For this review, take the finished solid that the model builds, in its own axes (mm). Round coordinates to 2 decimals unless told otherwise and drop trailing zeros. Order: outer loops, then holes, each group sorted by start corner. A loop starts at its lowest first (then second) coordinate and runs counter-clockwise, first axis right, second up. Notation, with made-up numbers: (86, -23) -> (94, -23) arc R29 cw to (94, 14) -> close; hole circle Ø5 at (32, -2.5). An arc over 180 degrees is marked (long way). Put each result on its own line as item: value. Start each with the question number.
```python
from build123d import *

# Parameters (mm, degrees)
F0_W     = 3
F0_H     = 22
F1_DEPTH = 3
F2_SIZE  = 2.99999


# Not quite as in the source:
# - a fillet or chamfer is up to 0.001 mm smaller than in the source, because OpenCascade refuses the exact size


with BuildPart() as f1:
    # F0 (on Top) → F1 (new body)
    with BuildSketch(Plane.XY):
        Polygon((-79.1548952963, 25), (-79.1548952963, 0), (118.8451047037, 0), (118.8451047037, 25), (118.8451047037, 47), (118.8451047037, 72), (-79.1548952963, 72), (-79.1548952963, 47), align=None)
        with Locations((120.3451047037, 36)):
            Rectangle(F0_W, F0_H)
        with Locations((-80.6548952963, 36)):
            Rectangle(F0_W, F0_H)
    extrude(amount=F1_DEPTH)

    # F2 (size 3 in the source; OpenCascade refuses exactly that, so slightly less here)
    f2_edges = [f1.edges().sort_by_distance(p)[0] for p in [
        (19.845105, 0, 3),
        (19.845105, 72, 3),
    ]]
    chamfer(f2_edges, length=F2_SIZE)


solid = f1.part
```
Item 1: Consider section B-B, the plane z = 1. Write out the cut boundary in (x, y).
Item 2: Consider section C-C, the plane y = 56. Write out the cut boundary in (x, z), plus the area to 3 significant figures.
Item 3: For L1, parallel to X at y = 11.5, z = 1.85; L2, parallel to Y at x = 39, z = 1.6; L3, parallel to Y at x = 29, z = 0.3, list the stretches that pass through material, from the lowest coordinate up.
Item 4: Insertion check: pin 1 Ø1.5 at (y, z) = (54, 1.5) entering from +X; pin 2 Ø0.9 at (x, z) = (-81, 1) entering from -Y; pin 3 Ø1 at (x, z) = (-30, 2.5) entering from -Y. Each pin has a flat end and moves straight along its axis. Give the tip position at first contact, or say it passes through.
Evaluation:
1. outline: (-82.15, 25) -> (-79.15, 25) -> (-79.15, 1) -> (118.85, 1) -> (118.85, 25) -> (121.85, 25) -> (121.85, 47) -> (118.85, 47) -> (118.85, 71) -> (-79.15, 71) -> (-79.15, 47) -> (-82.15, 47) -> close
2. outline: (-79.15, 0) -> (118.85, 0) -> (118.85, 3) -> (-79.15, 3) -> close
2. area: 594 mm^2
3. L1: x = -79.15 to 118.85
3. L2: y = 1.6 to 70.4
3. L3: y = 0.3 to 71.7
4. pin 1: stops at x = 118.85
4. pin 2: stops at y = 25
4. pin 3: stops at y = 2
